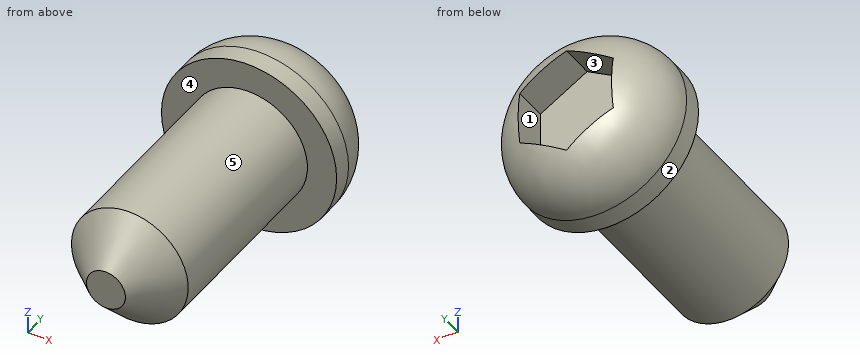
Autodesk Inventor part; units mm, degrees
ref_plane "Work Plane1" through (0, 6, 0) normal (0, 1, 0) x (1, 0, 0)
ref_plane "Work Plane2" through (0, 8, 0) normal (0, 1, 0) x (1, 0, 0)
ref_plane "YZ Plane" through (0, 0, 0) normal (1, 0, 0) x (0, 1, 0)
sketch "Sketch1" plane through (0, 0, 0) normal (0, 1, 0) x (-1, 0, 0)
  circle A0 centre (0, 0) radius 1.5
  dimension "d0" = 3
extrude "Extrusion1" add sketch "Sketch1" along normal blind 6
chamfer "Chamfer1" distance 1 angle 45 1 edges at (1.5, 0, 0)
ref_plane "Work Plane1" through (0, 6, 0) normal (0, 1, 0) x (1, 0, 0)
sketch "Sketch2" plane through (0, 6, 0) normal (0, 1, 0) x (1, 0, 0)
  circle A0 centre (0, 0) radius 0.5
  circle A1 centre (0, 0) radius 2.25
  dimension "d7" = 4.5
extrude "Extrusion2" add sketch "Sketch2" along normal blind 2 contours A0 | A1
fillet "Fillet1" radius 1.5 1 edges at (-2.25, 8, 0)
ref_plane "Work Plane2" through (0, 8, 0) normal (0, 1, 0) x (1, 0, 0)
sketch "Sketch3" plane through (0, 8, 0) normal (0, 1, 0) x (1, 0, 0)
  line L0 (-1.2, 0.6928) -> (0, 1.3856)
  line L1 (0, 1.3856) -> (1.2, 0.6928)
  line L2 (1.2, 0.6928) -> (1.2, -0.6928)
  line L3 (1.2, -0.6928) -> (0, -1.3856)
  line L4 (0, -1.3856) -> (-1.2, -0.6928)
  line L5 (-1.2, -0.6928) -> (-1.2, 0.6928)
  point P0 (0, 0)
  point P1 (0, 0)
  dimension "d12" = 1.2
extrude "Extrusion3" cut sketch "Sketch3" against normal blind 1
thread "Thread1"
properties part number "M3x6mm_screw"
Geometry: final body of the model. Coordinates: model frame, mm. Face numbers are marked on the shaded views. A direction names the side the tool comes from. Round coordinates to 2 decimals unless told otherwise and drop trailing zeros. Order: outer loops, then holes, each group sorted by start corner. A loop starts at its lowest first (then second) coordinate and runs counter-clockwise, first axis right, second up.
Q1. Access query for the marked faces 1 and 2. Directions: +Z, -Z, +X, -X, +Y, -Y. A direction counts if a zero-diameter tool reaches every point of the face in a straight line with its end or side. Return the directions, or none.
Result sheet:
face 1: +Y
face 2: +Y, -Y
Q2. Section A-A, the plane y = 4.5. Output: boundary loops of the cut face in (x, z).
Result sheet:
outline: circle Ø3 at (0, 0)
Q3. Mould query, pull axis X, two halves, no side actions, for the marked faces 3, 4 and 5. Classes: released by +X, released by -X, zero draft, split by the parting line, or undercut.
Result sheet:
face 3: undercut
face 4: zero draft
face 5: split by the parting line
Q4. Material intervals for probe 1 along Z at (x, y) = (-1.15, 7.25); probe 2 along X at (y, z) = (7.5, 1.1); probe 3 along Y at (x, z) = (1, 1), sorted ascending.
Result sheet:
probe 1: z = -1.7 to -0.72, 0.72 to 1.7
probe 2: x = -1.51 to -0.49, 0.49 to 1.51
probe 3: y = 0.91 to 7.84
Q5. Pin query (flat end, axial travel): pin 1 (0.5 mm diameter, centred on y = 7.5, z = 0.5, fed in from -X); pin 2 (2 mm diameter, centred on x = -1, z = 0, fed in from -Y); pin 3 (2 mm diameter, centred on x = -1.5, y = 2, fed in from -Z); pin 4 (0.5 mm diameter, centred on y = 7.5, z = 0, fed in from +X). Return the tip coordinate at first contact, or that it passes through.
Result sheet:
pin 1: stops at x = -2
pin 2: stops at y = 0
pin 3: stops at z = -1.41
pin 4: stops at x = 2.05
